Model file for the job. Use its own axes, mm. A direction names the side the tool comes from. Give positions to 0.01 mm unless a question says otherwise; leave off trailing zeros. Loops run counter-clockwise (first coordinate to the right, second up) from the corner with the lowest first, then second, coordinate; pieces in that order, holes last. Notation, with made-up numbers: (66.5, -17.5) -> (98.5, -17.5) arc R17 ccw to (98.5, -11.5) -> close; hole circle Ø1 at (85.5, 35.25). An arc over 180 degrees is marked (long way). Use CSV: the item, a comma, the result in double quotes. Start each with the question number.
(1) 3-axis set-ups, long thin cutter, end or side, ignore diameter. For faces 1 (the flat face through (7, -6, 45.8)), 2 (the flat face through (-3.76, -5.77, 43.12)), 3 (the flat face through (4, -5.7, 45.8)), 4 (the cylindrical face through (0, 2, 42)), 5 (the flat face through (-7, -6, 45.8)): which of +Z, -Z, +X, -X, +Y, -Y reach the whole face in a straight line?
(2) Pull direction X, two halves, no side cores. Call faces 6 (the flat face through (-6.856, -5.726, 45.011)), 7 (the flat face through (-4.36, -5.77, 44.99)), 8 (the flat face through (3.74, -5.73, 43.12)), 9 (the flat face through (7.444, -5.774, 43.115)): pulls with the +X half, pulls with the -X half, needs draft (parallel to the pull), parting line crosses it, or undercut.
(3) Cut at C-C on y = 2.25. Write the cut outline in (x, z), then the cut area to 3 significant figures.
(4) Cut at B-B on y = -6. Write the cut outline in (x, z), then the cut area to 3 significant figures.
(5) Cut at D-D on z = 30.5. Write the cut outline in (x, y).
(6) Flat gauge pins, fed straight in: pin 1 (1.2 mm diameter, centred on x = 7, y = -5, fed in from -Z); pin 2 (5 mm diameter, centred on y = 2.5, z = 15, fed in from +X); pin 3 (3 mm diameter, centred on y = 1.5, z = 26, fed in from -X). Where does each tip first touch, or does it go through?
(7) Cut at A-A on x = 0. Write the cut outline in (y, z), then the cut area to 3 significant figures.
(8) Drill centre lines: probe 1 along X at (y, z) = (-2.15, 45); probe 2 along Y at (x, z) = (2.25, 19); probe 3 along X at (y, z) = (2, 26). Where is each one in solid material? Low to high.
from build123d import *
from build123d.topology import SkipClean

# Parameters (mm, degrees)
EXTRUDE_1_DEPTH     = 4
EXTRUDE_3_DEPTH     = 6
CHAMFER_1_SIZE      = 3
CUT_EXTRUDE_2_DEPTH = 3.99
CUT_EXTRUDE_3_REACH = 51.222
SKETCH_7_R          = 1.5
SKETCH_8_R          = 6
EXTRUDE_4_DEPTH     = 1
FILLET_1_R          = 0.5
SKETCH_9_R          = 5
CUT_EXTRUDE_4_DEPTH = 3
SKETCH_10_R         = 3.55
CUT_EXTRUDE_5_DEPTH = 3.6
CUT_EXTRUDE_6_DEPTH = 0.8
CUT_EXTRUDE_7_DEPTH = 50.986598204
FILLET_2_R          = 2


with BuildPart() as part:
    # ｽｹｯﾁ1 → ﾎﾞｽ - 押し出し1 (new body)
    with BuildSketch(Plane(origin=(0, 0, 0), x_dir=(1, 0, 0), z_dir=(0, 1, 0))):
        with BuildLine():
            Line((-7.9, 0), (-7.9, -48))
            Line((-7.9, -48), (7.9, -48))
            Line((7.9, -48), (7.9, 0))
            ThreePointArc((7.9, 0), (0, 7.9), (-7.9, 0))
        make_face()
    extrude(amount=EXTRUDE_1_DEPTH)

    # ｽｹｯﾁ4 → ﾎﾞｽ - 押し出し3 (add)
    with BuildSketch(Plane.XY.offset(48)):
        Polygon((-7, -7.5), (-4.5, -7.5), (-3, -4), (3, -4), (4.5, -7.5), (7, -7.5), (7.9, -4), (7.9, 0), (-7.9, 0), (-7.9, -4), align=None)
    extrude(amount=-EXTRUDE_3_DEPTH)

    # 面取り1
    chamfer_1_edges = [part.edges().sort_by_distance(p)[0] for p in [
        (0, 4, 48),
    ]]
    chamfer(chamfer_1_edges, length=CHAMFER_1_SIZE)

    # ｽｹｯﾁ6 → ｶｯﾄ - 押し出し2 (cut)
    with BuildSketch(Plane(origin=(0, 4, 0), x_dir=(1, 0, 0), z_dir=(0, 1, 0))):
        with BuildLine():
            Line((-3, -45), (-3, -49))
            Line((-3, -49), (3, -49))
            Line((3, -49), (3, -45))
            ThreePointArc((3, -45), (0, -42), (-3, -45))
        make_face()
    extrude(amount=-CUT_EXTRUDE_2_DEPTH, mode=Mode.SUBTRACT)

    # ｽｹｯﾁ7 → ｶｯﾄ - 押し出し3 (cut, up to next)
    with BuildSketch(Plane(origin=(0, 0.01, 0), x_dir=(1, 0, 0), z_dir=(0, 1, 0)), mode=Mode.PRIVATE) as cut_extrude_3_sk1:
        with Locations(Location((0, -45, 0), (0, 0, 270))):
            Circle(SKETCH_7_R)
    cut_extrude_3_tool1 = extrude(cut_extrude_3_sk1.sketch, amount=-CUT_EXTRUDE_3_REACH, mode=Mode.PRIVATE) & part.part
    add(cut_extrude_3_tool1.solids().sort_by_distance((0, 0.01, 45))[0], mode=Mode.SUBTRACT)

    # ｽｹｯﾁ8 → ﾎﾞｽ - 押し出し4 (add)
    with BuildSketch(Plane.XZ):
        with Locations(Location((0, 0, 0), (0, 0, 90))):
            Circle(SKETCH_8_R)
    extrude(amount=EXTRUDE_4_DEPTH)

    # ﾌｨﾚｯﾄ1
    fillet_1_edges = [part.edges().sort_by_distance(p)[0] for p in [
        (0, 0, -6),
    ]]
    fillet(fillet_1_edges, radius=FILLET_1_R)

    # ｽｹｯﾁ9 → ｶｯﾄ - 押し出し4 (cut)
    with BuildSketch(Plane(origin=(0, 4, 0), x_dir=(1, 0, 0), z_dir=(0, 1, 0))):
        with Locations(Location((0, 0, 0), (0, 0, 270))):
            Circle(SKETCH_9_R)
    extrude(amount=-CUT_EXTRUDE_4_DEPTH, mode=Mode.SUBTRACT)

    # ｽｹｯﾁ10 → ｶｯﾄ - 押し出し5 (cut)
    with BuildSketch(Plane(origin=(0, 1, 0), x_dir=(1, 0, 0), z_dir=(0, 1, 0))):
        with Locations(Location((0, 0, 0), (0, 0, 270))):
            Circle(SKETCH_10_R)
    extrude(amount=-CUT_EXTRUDE_5_DEPTH, mode=Mode.SUBTRACT)

    # ｽｹｯﾁ11 → ｶｯﾄ - 押し出し6 (cut, symmetric)
    with BuildSketch(Plane.XY.offset(45)):
        Polygon((3, -4), (4.5, -7.5), (5.1, -7.5), (3.6, -4), align=None)
        Polygon((6.4, -7.5), (7, -7.5), (7.9, -4), (7.3, -4), align=None)
    cut_extrude_6 = extrude(amount=CUT_EXTRUDE_6_DEPTH, both=True, mode=Mode.SUBTRACT)

    # ﾐﾗｰ1: ｶｯﾄ - 押し出し6 across plane
    add(cut_extrude_6.mirror(Plane(origin=(0, 0, 0), x_dir=(0, 0, 1), z_dir=(1, 0, 0))), mode=Mode.SUBTRACT)

    # ｽｹｯﾁ12 → ｶｯﾄ - 押し出し7 (cut, through all)
    with SkipClean():  # the faces are left unmerged after this step: merging them gives an invalid solid
        with BuildSketch(Plane(origin=(0, 4, 0), x_dir=(1, 0, 0), z_dir=(0, 1, 0))):
            with BuildLine():
                Line((-7.9, 0), (-7.9, -40))
                Line((-7.9, -40), (-6.9, -37))
                Line((-6.9, -37), (-6.9, -3.847076812))
                ThreePointArc((-6.9, -3.847076812), (-7.645913941, -1.987460691), (-7.9, 0))
            make_face()
        cut_extrude_7 = extrude(amount=-CUT_EXTRUDE_7_DEPTH, mode=Mode.SUBTRACT)

    # ﾐﾗｰ2: ｶｯﾄ - 押し出し7 across plane
    with SkipClean():  # the faces are left unmerged after this step: merging them gives an invalid solid
        add(cut_extrude_7.mirror(Plane(origin=(0, 0, 0), x_dir=(0, 0, 1), z_dir=(1, 0, 0))), mode=Mode.SUBTRACT)

    # ﾌｨﾚｯﾄ2
    fillet_2_edges = [part.edges().sort_by_distance(p)[0] for p in [
        (-6.9, 2, 3.847076812),
        (-6.9, 2, 37),
        (-7.9, 2, 40),
        (6.9, 2, 3.847076812),
        (7.9, 2, 40),
        (6.9, 2, 37),
    ]]
    fillet(fillet_2_edges, radius=FILLET_2_R)

    # Surface Cut 1
    split(bisect_by=Plane.XY.offset(8), keep=Keep.TOP)


solid = part.part
Check result:
1,face 1,"+X, -Y"
1,face 2,"+Z, -Z, -Y"
1,face 3,"-Y"
1,face 4,"+Z, +Y"
1,face 5,"-X, -Y"
2,face 6,"pulls with the -X half"
2,face 7,"undercut"
2,face 8,"undercut"
2,face 9,"pulls with the +X half"
3,outline,"(-7.9, 40.32) arc R2 ccw to (-7.8, 39.69) -> (-7, 37.31) arc R2 cw to (-6.9, 36.68) -> (-6.9, 8) -> (6.9, 8) -> (6.9, 36.68) arc R2 cw to (7, 37.31) -> (7.8, 39.69) arc R2 ccw to (7.9, 40.32) -> (7.9, 46.75) -> (3, 46.75) -> (3, 45) arc R3 cw to (-3, 45) -> (-3, 46.75) -> (-7.9, 46.75) -> close"
3,area,"527 mm²"
4,outline,"(-7.39, 42) -> (-3.86, 42) -> (-3.86, 44.2) -> (-4.46, 44.2) -> (-4.46, 45.8) -> (-3.86, 45.8) -> (-3.86, 48) -> (-7.39, 48) -> (-7.39, 45.8) -> (-6.79, 45.8) -> (-6.79, 44.2) -> (-7.39, 44.2) -> close; (3.86, 42) -> (7.39, 42) -> (7.39, 44.2) -> (6.79, 44.2) -> (6.79, 45.8) -> (7.39, 45.8) -> (7.39, 48) -> (3.86, 48) -> (3.86, 45.8) -> (4.46, 45.8) -> (4.46, 44.2) -> (3.86, 44.2) -> close"
4,area,"38.5 mm²"
5,outline,"(-6.9, 0) -> (6.9, 0) -> (6.9, 4) -> (-6.9, 4) -> close"
6,pin 1,"z = 42"
6,pin 2,"x = 6.9"
6,pin 3,"x = -6.9"
7,outline,"(-4, 42) -> (0, 42) -> (0, 8) -> (4, 8) -> (4, 42) -> (0.01, 42) -> (0.01, 43.5) -> (-4, 43.5) -> close; (-4, 46.5) -> (0.01, 46.5) -> (0.01, 48) -> (-4, 48) -> close"
7,area,"148 mm²"
8,probe 1,"-7.9 to -1.5, 1.5 to 7.9"
8,probe 2,"0 to 4"
8,probe 3,"-6.9 to 6.9"
